```python
from build123d import *

# Parameters (mm, degrees)
SKETCH2_R           = 85
SKETCH2_R_2         = 20
BOSS_EXTRUDE1_DEPTH = 10
CUT_EXTRUDE1_START  = -5
CUT_EXTRUDE1_DEPTH  = 5


with BuildPart() as part:
    # Sketch2 → Boss-Extrude1 (new body)
    with BuildSketch(Plane.XY):
        Circle(SKETCH2_R)
        Circle(SKETCH2_R_2, mode=Mode.SUBTRACT)
    extrude(amount=BOSS_EXTRUDE1_DEPTH)

    # Sketch3 → Cut-Extrude1 (cut)
    with BuildSketch(Plane.XY.offset(10).offset(CUT_EXTRUDE1_START)):
        with BuildLine():
            Line((-18.33030278, 8), (-84.622691992, 8))
            ThreePointArc((-84.622691992, 8), (-85, 0), (-84.622691992, -8))
            Line((-84.622691992, -8), (-18.33030278, -8))
            ThreePointArc((-18.33030278, -8), (-20, 0), (-18.33030278, 8))
        make_face()
        with BuildLine():
            ThreePointArc((85, 0), (84.905620601, 4.00444632), (84.622691992, 8))
            Line((84.622691992, 8), (18.33030278, 8))
            ThreePointArc((18.33030278, 8), (19.578126259, 4.086192874), (20, 0))
            ThreePointArc((20, 0), (19.578126259, -4.086192874), (18.33030278, -8))
            Line((18.33030278, -8), (84.622691992, -8))
            ThreePointArc((84.622691992, -8), (84.905620601, -4.00444632), (85, 0))
        make_face()
        with BuildLine():
            ThreePointArc((8, 84.622691992), (0, 85), (-8, 84.622691992))
            Line((-8, 84.622691992), (-8, 18.33030278))
            ThreePointArc((-8, 18.33030278), (0, 20), (8, 18.33030278))
            Line((8, 18.33030278), (8, 84.622691992))
        make_face()
        with BuildLine():
            Line((-8, -18.33030278), (-8, -84.622691992))
            ThreePointArc((-8, -84.622691992), (0, -85), (8, -84.622691992))
            Line((8, -84.622691992), (8, -18.33030278))
            ThreePointArc((8, -18.33030278), (0, -20), (-8, -18.33030278))
        make_face()
    extrude(amount=CUT_EXTRUDE1_DEPTH, mode=Mode.SUBTRACT)


solid = part.part
```
Read the model definition and answer for the solid it produces. Units are mm, in the model's axes. A direction names the side the tool comes from. Coordinates: 2 decimals unless noted, no trailing zeros. Write each loop counter-clockwise with the first axis right and the second up, starting at its lowest first coordinate (ties: lowest second). Pieces come first, ordered by that corner, then holes. Notation, with made-up numbers: (-2.75, 1.5) -> (30.25, 1.5) arc R23 ccw to (30.25, 10.5) -> close; hole circle Ø9 at (30, 59.25). An arc over 180 degrees is marked (long way). Answer as a JSON object with one key per item and string values.
Q1. The part is cut by section B-B on x = 0. Give the vertices of the cut face in (y, z).
The answers:
{"outline": "(-85, 0) -> (-20, 0) -> (-20, 5) -> (-85, 5) -> close; (20, 0) -> (85, 0) -> (85, 5) -> (20, 5) -> close"}
Q2. The part is cut by section D-D on y = 70. Give the vertices of the cut face in (x, z).
The answers:
{"outline": "(-48.22, 0) -> (48.22, 0) -> (48.22, 10) -> (8, 10) -> (8, 5) -> (-8, 5) -> (-8, 10) -> (-48.22, 10) -> close"}
Q3. Determine the mould class of faces 4 (the flat face through (-38, 38, 10)), 5 (the cylindrical face through (-19.98, 0.88, 3.82)), 6 (the cylindrical face through (81.075, 25.532, 4.93)) for opening direction Y: pulls with the +Y half, pulls with the -Y half, needs draft (parallel to the pull), parting line crosses it, or undercut.
The answers:
{"face 4": "needs draft", "face 5": "undercut", "face 6": "parting line crosses it"}
Q4. The part is cut by section A-A on z = 6.5. Give the vertices of the cut face in (x, y), then the cut area to 3 significant figures.
The answers:
{"outline": "(-84.62, -8) arc R85 ccw to (-8, -84.62) -> (-8, -18.33) arc R20 cw to (-18.33, -8) -> close; (-84.62, 8) -> (-18.33, 8) arc R20 cw to (-8, 18.33) -> (-8, 84.62) arc R85 ccw to start; (8, -84.62) arc R85 ccw to (84.62, -8) -> (18.33, -8) arc R20 cw to (8, -18.33) -> close; (8, 18.33) arc R20 cw to (18.33, 8) -> (84.62, 8) arc R85 ccw to (8, 84.62) -> close", "area": "17,300 mm2"}
Q5. Consider line 1 (X direction, y = 75, z = 7); line 2 (Y direction, x = -17, z = 7.5); line 3 (X direction, y = 43, z = 5.5). Determine where each line is inside the solid, lowest interval first. Write a range as [from, to].
The answers:
{"line 1": "x = [-40, -8], [8, 40]", "line 2": "y = [-83.28, -10.54], [10.54, 83.28]", "line 3": "x = [-73.32, -8], [8, 73.32]"}
Q6. Flat-ended cylindrical pins translate along their axes: pin 1 Ø13 at (x, y) = (-2.5, 42.5) entering from +Z; pin 2 Ø2.5 at (y, z) = (-46, 8) entering from +X; pin 3 Ø6 at (y, z) = (-55, 1.5) entering from +X; pin 4 Ø2.5 at (y, z) = (41.5, 8) entering from -X. Find the tip coordinate at first contact, or state that the pin passes through.
The answers:
{"pin 1": "stops at z = 10", "pin 2": "stops at x = 72.27", "pin 3": "stops at x = 67.24", "pin 4": "stops at x = -74.87"}
Q7. A tool of negligible diameter and unlimited length cuts with its end or side. For faces 1 (the flat face through (8, -52, 7)), 2 (the flat face through (37, -37, 10)), 3 (the flat face through (-52, -8, 7)), from which of +Z, -Z, +X, -X, +Y, -Y can it reach the whole face along a straight path? Write none if from no direction.
The answers:
{"face 1": "+Z, +Y, -Y", "face 2": "+Z, +X, -X, +Y, -Y", "face 3": "+Z, +X, -X"}
